Read the model definition and answer for the solid it produces. Units are mm, in the model's axes. Coordinates: 2 decimals unless noted, no trailing zeros. Write each loop counter-clockwise with the first axis right and the second up, starting at its lowest first coordinate (ties: lowest second). Pieces come first, ordered by that corner, then holes. Notation, with made-up numbers: (-4, 5.25) -> (6, 5.25) arc R15 cw to (6, 14.25) -> close; hole circle Ø4 at (56, 24.5). An arc over 180 degrees is marked (long way). Return JSON: item names as keys, results as strings.
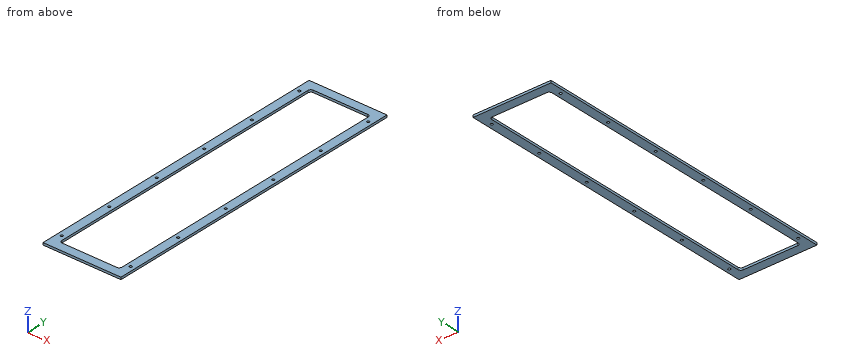
from build123d import *

# Parameters (mm, degrees)
SKETCH002_W            = 140
SKETCH002_H            = 560
PAD001_DEPTH           = 4
SKETCH003_R            = 2.2
POCKET001_DEPTH        = 4.001
LINEARPATTERN001_COUNT = 6
LINEARPATTERN001_PITCH = 100


with BuildPart() as part:
    # Sketch002 → Pad001 (new body)
    with BuildSketch(Plane.XY):
        with Locations((0, 280)):
            Rectangle(SKETCH002_W, SKETCH002_H)
        with BuildLine():
            Line((-49, 544), (49, 544))
            ThreePointArc((54, 539), (52.535534, 542.535534), (49, 544))
            Line((54, 539), (54, 21))
            ThreePointArc((49, 16), (52.535534, 17.464466), (54, 21))
            Line((49, 16), (-49, 16))
            ThreePointArc((-54, 21), (-52.535534, 17.464466), (-49, 16))
            Line((-54, 21), (-54, 539))
            ThreePointArc((-49, 544), (-52.535534, 542.535534), (-54, 539))
        make_face(mode=Mode.SUBTRACT)
    extrude(amount=PAD001_DEPTH)

    # Sketch003 (on Face14 of Pad001) → Pocket001 (cut, through all)
    with BuildSketch(Plane.XY.offset(4)):
        with Locations((62, 30)):
            Circle(SKETCH003_R)
        with Locations((-62, 30)):
            Circle(SKETCH003_R)
    pocket001 = extrude(amount=-POCKET001_DEPTH, mode=Mode.SUBTRACT)

    # LinearPattern001: Pocket001 ×6
    with Locations(*[(0, i * LINEARPATTERN001_PITCH, 0) for i in range(1, LINEARPATTERN001_COUNT)]):
        add(pocket001, mode=Mode.SUBTRACT)


with BuildPart() as part_1:
    # Body001 placement: moved
    add(part.part.moved(Location((0, 0, 40))))


solid = part_1.part
1. The part is cut by section C-C (z = 40.8). Count the separate pieces of the cut face and the enclosed holes in it, then the cut area to 3 significant figures.
Taken from the geometry:
{"separate pieces": "1", "enclosed holes": "13", "area": "21,200 mm2"}
2. Consider L1, parallel to X at y = 130, z = 40.95; L2, parallel to X at y = 484.5, z = 42.3; L3, parallel to Y at x = -3.5, z = 43.35. Determine where each line is inside the solid, lowest interval first.
Taken from the geometry:
{"L1": "x = -70 to -64.2, -59.8 to -54, 54 to 59.8, 64.2 to 70", "L2": "x = -70 to -54, 54 to 70", "L3": "y = 0 to 16, 544 to 560"}
3. The part is cut by section A-A (x = 13). Determine the outline of the cut face in (y, z), then the cut area to 3 significant figures.
Taken from the geometry:
{"outline": "(0, 40) -> (16, 40) -> (16, 44) -> (0, 44) -> close; (544, 40) -> (560, 40) -> (560, 44) -> (544, 44) -> close", "area": "128 mm2"}
4. The part is cut by section B-B (y = 391). Determine the outline of the cut face in (x, z), then the cut area to 3 significant figures.
Taken from the geometry:
{"outline": "(-70, 40) -> (-54, 40) -> (-54, 44) -> (-70, 44) -> close; (54, 40) -> (70, 40) -> (70, 44) -> (54, 44) -> close", "area": "128 mm2"}
